Could you check a few things on this model? Use its own coordinates, in mm. Face numbers are marked on the shaded views. Coordinates: 2 decimals unless noted, no trailing zeros. Order: outer loops, then holes, each group sorted by start corner. A loop starts at its lowest first (then second) coordinate and runs counter-clockwise, first axis right, second up.
```python
from build123d import *

# Parameters (mm, degrees)
SKETCH1_W              = 31.75
SKETCH1_H              = 12.7
BOSS_EXTRUDE1_DEPTH    = 6.35
SKETCH2_R              = 2.5527
CUT_EXTRUDE1_DEPTH     = 37.477972806
F_10_32_TAPPED_HOLE1_D = 4.0386


with BuildPart() as part:
    # Sketch1 → Boss-Extrude1 (new, symmetric)
    with BuildSketch(Plane.XY):
        with Locations((15.875, 6.35)):
            Rectangle(SKETCH1_W, SKETCH1_H)
    extrude(amount=BOSS_EXTRUDE1_DEPTH, both=True)

    # Sketch2 → Cut-Extrude1 (cut, through all)
    with BuildSketch(Plane.XY.offset(6.35)):
        with Locations((4.7625, 6.35)):
            Circle(SKETCH2_R)
        with Locations((26.9875, 6.35)):
            Circle(SKETCH2_R)
    extrude(amount=-CUT_EXTRUDE1_DEPTH, mode=Mode.SUBTRACT)

    # #10-32 Tapped Hole1 (through all)
    with Locations(Plane(origin=(15.875, 12.7, 0), x_dir=(0, 0, 1), z_dir=(0, 1, 0))):
        with Locations((0, 0)):
            Hole(F_10_32_TAPPED_HOLE1_D / 2)


solid = part.part
```
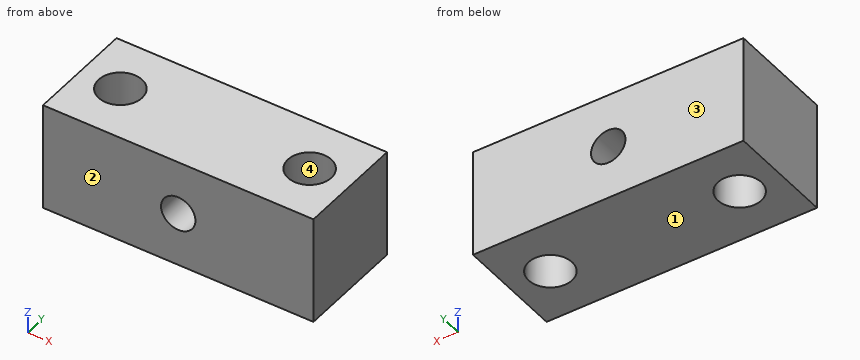
Item 1: Suppose I cut it at C-C (x = 25). List the corners of the cut face in (y, z) for me, and give its area (3 significant figures).
Item 2: Suppose I cut it at D-D (y = 1.5). List the corners of the cut face in (x, z) for me (3 decimals), and give its area (3 significant figures).
Item 3: Suppose I cut it at B-B (y = 4.5). List the corners of the cut face in (x, z) for me (3 decimals).
Item 4: Thinking about a two-plate mould opening in Y: for the marked faces 1, 2, 3 and 4, which applies, +Y half, -Y half, draft (parallel to the pull), parting line (faces both ways), or undercut?
Item 5: For pin 1 Ø3.5 at (x, z) = (15.875, 0) entering from +Y; pin 2 Ø1.5 at (y, z) = (5.5, -1.5) entering from -X, each with a flat end and sliding along its axis, tell me the tip position at first contact or that it passes through.
Item 6: Suppose I cut it at A-A (z = 0). List the corners of the cut face in (x, y) for me.
Item 7: I need wall thicknesses on line 1 (X direction, y = 4.5, z = 0.25); line 2 (X direction, y = 7.25, z = -4.25); line 3 (X direction, y = 10.5, z = 0.75). Which ranges of each line are inside material? Lowest first, please.
Geometry results:
1. outline: (0, -6.35) - (4.75, -6.35) - (4.75, 6.35) - (0, 6.35) - close; (7.95, -6.35) - (12.7, -6.35) - (12.7, 6.35) - (7.95, 6.35) - close
1. area: 121 mm2
2. outline: (0, -6.35) - (31.75, -6.35) - (31.75, 6.35) - (0, 6.35) - close; hole circle Ø4.039 at (15.875, 0)
2. area: 390 mm2
3. outline: (0, -6.35) - (3.004, -6.35) - (3.004, 6.35) - (0, 6.35) - close; (6.521, -6.35) - (25.229, -6.35) - (25.229, 6.35) - (6.521, 6.35) - close; (28.746, -6.35) - (31.75, -6.35) - (31.75, 6.35) - (28.746, 6.35) - close; hole circle Ø4.039 at (15.875, 0)
4. face 1: draft
4. face 2: -Y half
4. face 3: +Y half
4. face 4: undercut
5. pin 1: passes through
5. pin 2: stops at x = 0
6. outline: (0, 0) - (13.86, 0) - (13.86, 12.7) - (0, 12.7) - close; (17.89, 0) - (31.75, 0) - (31.75, 12.7) - (17.89, 12.7) - close; hole circle Ø5.11 at (4.76, 6.35); hole circle Ø5.11 at (26.99, 6.35)
7. line 1: x = 0 to 3, 6.52 to 13.87, 17.88 to 25.23, 28.75 to 31.75
7. line 2: x = 0 to 2.37, 7.15 to 24.6, 29.38 to 31.75
7. line 3: x = 0 to 14, 17.75 to 31.75
